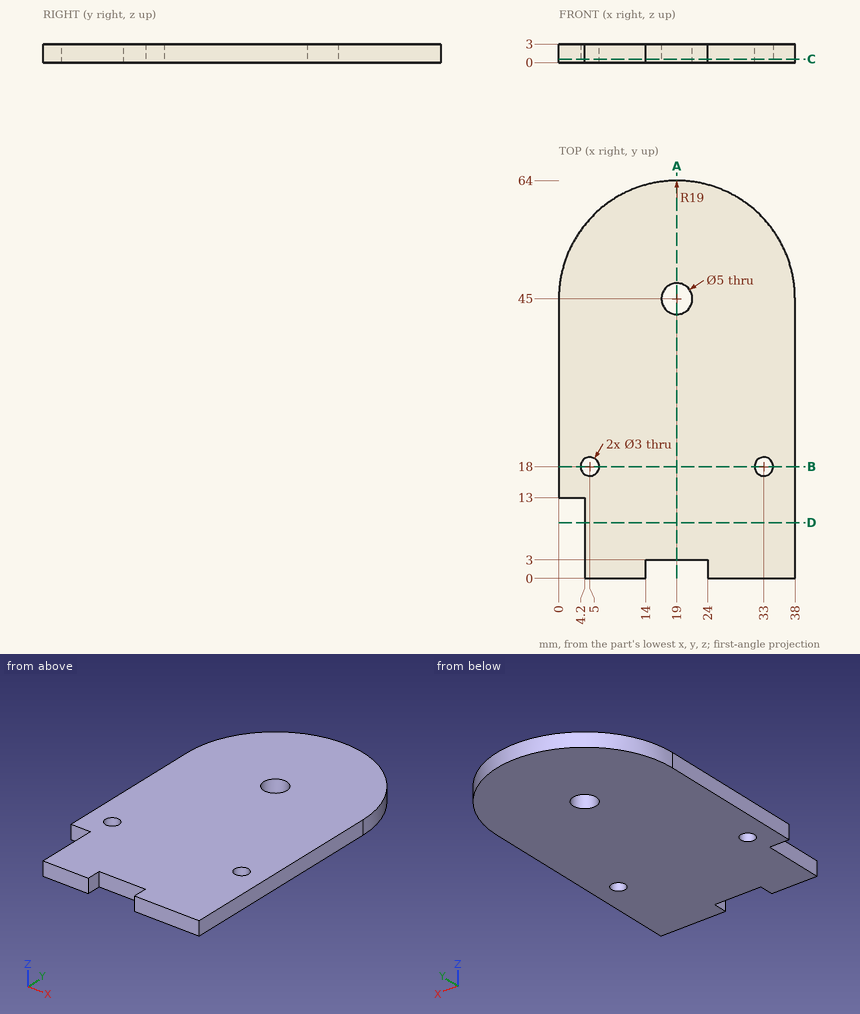
Input: dimensioned drawing with shaded views. Units: mm. Origin: part minimum x, y, z. Give positions to 0.01 mm unless a question says otherwise; leave off trailing zeros. Write each loop counter-clockwise with the first axis right and the second up, starting at its lowest first coordinate (ties: lowest second). Pieces come first, ordered by that corner, then holes. Notation, with made-up numbers: (-9, 74) -> (31, 74) arc R27 ccw to (31, 103) -> close; hole circle Ø1 at (52, 67.25). An arc over 180 degrees is marked (long way). Answer as a JSON object with one key per item and string values.
1. Cut plane C-C on z = 0.55. Output: boundary loops of the cut face in (x, y).
Ans:
{"outline": "(0, 13) -> (4.2, 13) -> (4.2, 0) -> (14, 0) -> (14, 3) -> (24, 3) -> (24, 0) -> (38, 0) -> (38, 45) arc R19 ccw to (0, 45) -> close; hole circle Ø3 at (5, 18); hole circle Ø5 at (19, 45); hole circle Ø3 at (33, 18)"}
2. Ray query, probe 1 along Y at (x, z) = (4, 2.45); probe 2 along Y at (x, z) = (19, 1.6); probe 3 along X at (y, z) = (43, 0.1). Return the intervals inside material, ascending. Write a range as from..to.
Ans:
{"probe 1": "y = 13..16.88, 19.12..56.66", "probe 2": "y = 3..42.5, 47.5..64", "probe 3": "x = 0..17.5, 20.5..38"}
3. Contact query for flat-ended pins moving along their axis: pin 1 (1.5 mm diameter, centred on y = 2, z = 2, fed in from -X); pin 2 (1.5 mm diameter, centred on x = 28, z = 0.5, fed in from +Y). Output: stop coordinate, or through.
Ans:
{"pin 1": "stops at x = 4.2", "pin 2": "stops at y = 62.12"}
4. Cut plane B-B on y = 18. Output: boundary loops of the cut face in (x, z).
Ans:
{"outline": "(0, 0) -> (3.5, 0) -> (3.5, 3) -> (0, 3) -> close; (6.5, 0) -> (31.5, 0) -> (31.5, 3) -> (6.5, 3) -> close; (34.5, 0) -> (38, 0) -> (38, 3) -> (34.5, 3) -> close"}
5. Cut plane A-A on x = 19. Output: boundary loops of the cut face in (y, z).
Ans:
{"outline": "(3, 0) -> (42.5, 0) -> (42.5, 3) -> (3, 3) -> close; (47.5, 0) -> (64, 0) -> (64, 3) -> (47.5, 3) -> close"}
6. Cut plane D-D on y = 9. Output: boundary loops of the cut face in (x, z), and give its area (3 significant figures).
Ans:
{"outline": "(4.2, 0) -> (38, 0) -> (38, 3) -> (4.2, 3) -> close", "area": "101 mm^2"}
